Verification items for the finished model (mm, model axes). A direction names the side the tool comes from. Round coordinates to 2 decimals unless told otherwise and drop trailing zeros. Write each loop counter-clockwise with the first axis right and the second up, starting at its lowest first coordinate (ties: lowest second). Pieces come first, ordered by that corner, then holes. Notation, with made-up numbers: (-2.75, 59.5) - (37.25, 59.5) arc R8 ccw to (37.25, 67.5) - close; hole circle Ø4 at (-18.5, 73.25). An arc over 180 degrees is marked (long way). Write each question's results on one line, items separated by ' | '.
```python
from build123d import *

# Parameters (mm, degrees)
SKETCH_1_W = 2.5
SKETCH_1_H = 3


with BuildPart() as part:
    # 草图1 → 旋转1 (revolve)
    with BuildSketch(Plane.XY, mode=Mode.PRIVATE) as revolve_1_sk:
        with Locations((1.25, 1.5)):
            Rectangle(SKETCH_1_W, SKETCH_1_H)
        Polygon((3, 0), (3, 3.5), (2.5, 3.5), (2.5, 3), (2.5, 0), align=None)
        Polygon((3.5, 0), (3, 0), (3, 3.5), align=None)
    revolve_1 = revolve(revolve_1_sk.sketch.rotate(Axis((0, 0, 0), (1, 0, 0)), 90), axis=Axis((0, 0, 0), (1, 0, 0)))

    # 镜向1: 旋转1 across plane
    add(revolve_1.mirror(Plane.ZY))


solid = part.part
```
(1) Go/stop test with flat-tipped pins: pin 1 Ø2 at (x, y) = (-1, 0) entering from -Z; pin 2 Ø1.5 at (x, y) = (-0.5, 2) entering from +Z; pin 3 Ø2 at (y, z) = (-1, -0.5) entering from +X. Record where each tip stops, or that it passes through.
Answer:
pin 1: z = -3 | pin 2: z = 2.73 | pin 3: x = 3.48
(2) Thickness scan on L1, parallel to X at y = -2.75, z = -1.5; L2, parallel to X at y = -1.75, z = 2.75; L3, parallel to Y at x = -0.5, z = 0. Record the ranges inside material, lowest first.
Answer:
L1: -3.05 to -2.5, 2.5 to 3.05 | L2: -3.03 to -2.5, 2.5 to 3.03 | L3: -3 to 3
(3) Mould release check, pull along X, two halves, no side actions. Record for faces 3 (the cylindrical face through (2.746, 3.105, 1.615)), 4 (the cylindrical face through (-0.04, -0.9, 2.86)), 5 (the conical face through (-3.476, 0.166, -0.037)): released by +X, released by -X, zero draft, split by the parting line, or undercut.
Answer:
face 3: zero draft | face 4: undercut | face 5: released by -X
(4) Set-up check for faces 1 (the cylindrical face through (-2.746, 3.105, 1.615)), 2 (the flat face through (2.5, -1, 3)): record each of +Z, -Z, +X, -X, +Y, -Y from which the full face is reachable in a straight line by a thin tool's end or side.
Answer:
face 1: +X, -X | face 2: none
(5) Section check A-A (x = -2). Record the cut outline in (y, z).
Answer:
outline: circle Ø6 at (0, 0)
